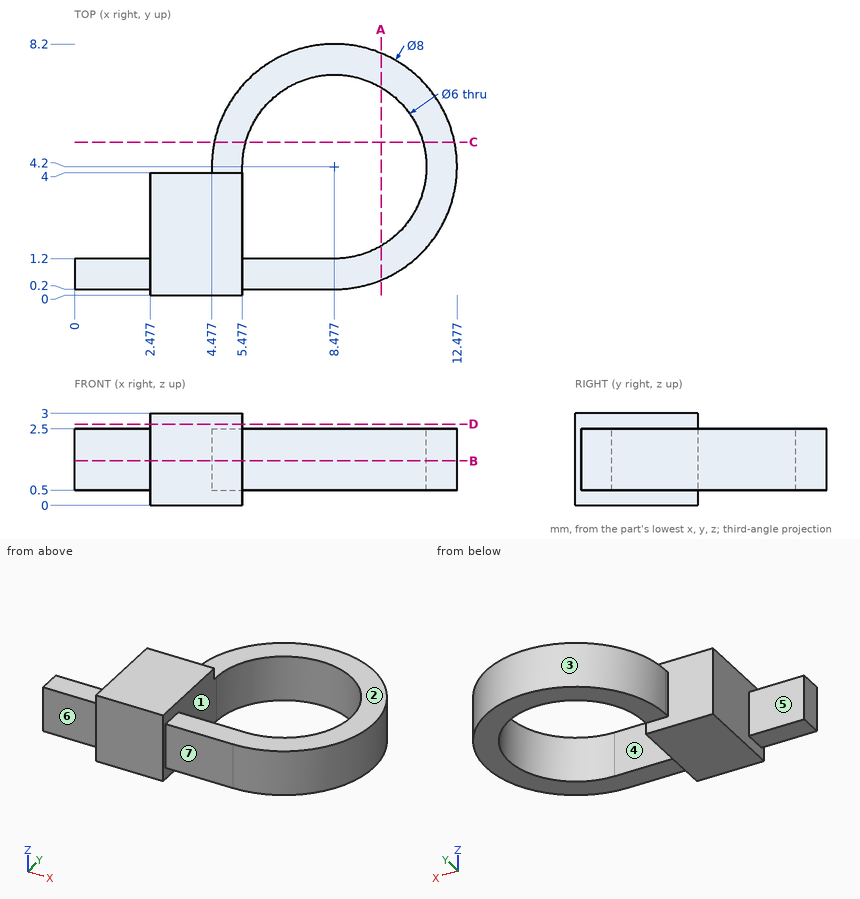
Input: dimensioned drawing with shaded views. Units: mm. Origin: part minimum x, y, z. A direction names the side the tool comes from. Round coordinates to 2 decimals unless told otherwise and drop trailing zeros. Order: outer loops, then holes, each group sorted by start corner. A loop starts at its lowest first (then second) coordinate and runs counter-clockwise, first axis right, second up.
Q1. Section B-B, the plane z = 1.45. Output: boundary loops of the cut face in (x, y).
Result sheet:
outline: (0, 0.2) - (2.48, 0.2) - (2.48, 0) - (5.48, 0) - (5.48, 0.2) - (8.48, 0.2) arc R4 ccw (long way) to (4.48, 4.2) - (4.48, 4) - (2.48, 4) - (2.48, 1.2) - (0, 1.2) - close; hole (5.48, 1.2) - (8.48, 1.2) arc R3 ccw (long way) to (5.48, 4.2) - close
Q2. Section C-C, the plane y = 5. Output: boundary loops of the cut face in (x, z) (1 decimal).
Result sheet:
outline: (4.6, 0.5) - (5.6, 0.5) - (5.6, 2.5) - (4.6, 2.5) - close; (11.4, 0.5) - (12.4, 0.5) - (12.4, 2.5) - (11.4, 2.5) - close
Q3. Mould query, pull axis X, two halves, no side actions, for the marked faces 1, 2 and 3. Classes: released by +X, released by -X, zero draft, split by the parting line, or undercut.
Result sheet:
face 1: undercut
face 2: zero draft
face 3: split by the parting line
Q4. Pin query (flat end, axial travel): pin 1 (1 mm diameter, centred on y = 3.5, z = 1, fed in from -X); pin 2 (0.9 mm diameter, centred on y = 2, z = 2, fed in from +X); pin 3 (0.6 mm diameter, centred on x = 1.5, z = 1, fed in from +Y). Return the tip coordinate at first contact, or that it passes through.
Result sheet:
pin 1: stops at x = 2.48
pin 2: stops at x = 12.07
pin 3: stops at y = 1.2
Q5. Section A-A, the plane x = 10. Output: boundary loops of the cut face in (y, z) (1 decimal).
Result sheet:
outline: (0.5, 0.5) - (1.6, 0.5) - (1.6, 2.5) - (0.5, 2.5) - close; (6.8, 0.5) - (7.9, 0.5) - (7.9, 2.5) - (6.8, 2.5) - close
Q6. Material intervals for probe 1 along Y at (x, z) = (8.5, 0.9); probe 2 along Z at (x, y) = (9, 7.5); probe 3 along Y at (x, z) = (3.25, 1.5), sorted ascending.
Result sheet:
probe 1: y = 0.2 to 1.2, 7.2 to 8.2
probe 2: z = 0.5 to 2.5
probe 3: y = 0 to 4
Q7. Access query for the marked faces 4, 5, 6 and 7. Directions: +Z, -Z, +X, -X, +Y, -Y. A direction counts if a zero-diameter tool reaches every point of the face in a straight line with its end or side. Return the directions, or none.
Result sheet:
face 4: +Z, -Z
face 5: +Z, -Z, -X, +Y
face 6: +Z, -Z, -X, -Y
face 7: +Z, -Z, +X, -Y
Q8. Section D-D, the plane z = 2.65. Output: boundary loops of the cut face in (x, y), and give its area (3 significant figures).
Result sheet:
outline: (2.48, 0) - (5.48, 0) - (5.48, 4) - (2.48, 4) - close
area: 12.0 mm2
